Read the model definition and answer for the solid it produces. Units are mm, in the model's axes. A direction names the side the tool comes from. Coordinates: 2 decimals unless noted, no trailing zeros. Order: outer loops, then holes, each group sorted by start corner. A loop starts at its lowest first (then second) coordinate and runs counter-clockwise, first axis right, second up. Notation, with made-up numbers: (29, 33) -> (72, 33) arc R28 ccw to (72, 52) -> close; hole circle Ø7 at (30.25, -19). An arc over 180 degrees is marked (long way). Answer in a Markdown table with one row per item.
from build123d import *

# Parameters (mm, degrees)
SKETCH100_R             = 17.579923
SKETCH100_R_2           = 1.617669
PAD044_DEPTH            = 8
SKETCH101_W             = 5
SKETCH101_H             = 3
SKETCH102_R             = 12.788983
SKETCH102_R_2           = 6.518589
POCKET072_DEPTH         = 2
SKETCH103_W             = 7.319854
SKETCH103_H             = 4.413105
POCKET073_DEPTH         = 8.001
POCKET075_DEPTH         = 108.636829
POLARPATTERN003_COUNT   = 7
SKETCH112_R             = 2
POCKET079_DEPTH         = 17
BODY019_PLACEMENT_ANGLE = 180


with BuildPart() as part:
    # Sketch100 → Pad044 (new body)
    with BuildSketch(Plane.YZ):
        Circle(SKETCH100_R)
        Circle(SKETCH100_R_2, mode=Mode.SUBTRACT)
    extrude(amount=PAD044_DEPTH)

    # Sketch101 → Groove003 (revolve, cut)
    with BuildSketch(Plane.XY):
        with Locations((4, 16.079923)):
            Rectangle(SKETCH101_W, SKETCH101_H)
    revolve(axis=Axis((0, 0, 0), (1, 0, 0)), mode=Mode.SUBTRACT)

    # Sketch102 (on Face6 of Groove003) → Pocket072 (cut)
    with BuildSketch(Plane.YZ.offset(8)):
        Circle(SKETCH102_R)
        Circle(SKETCH102_R_2, mode=Mode.SUBTRACT)
    extrude(amount=-POCKET072_DEPTH, mode=Mode.SUBTRACT)

    # Sketch103 (on Face11 of Pocket072) → Pocket073 (cut, through all)
    with BuildSketch(Plane.YZ.offset(8)):
        with Locations((-0.062492, 19.721895)):
            Rectangle(SKETCH103_W, SKETCH103_H)
    extrude(amount=-POCKET073_DEPTH, mode=Mode.SUBTRACT)

    # Sketch105 → Pocket075 (cut, through all)
    with BuildSketch(Plane.YZ.offset(8)):
        with BuildLine():
            ThreePointArc((4.568379, 12.912664), (0, 13.69697), (-4.568379, 12.912664))
            Line((-4.568379, 12.912664), (0, 5))
            Line((4.568379, 12.912664), (0, 5))
        make_face()
    pocket075 = extrude(amount=-POCKET075_DEPTH, mode=Mode.SUBTRACT)

    # PolarPattern003: Pocket075 ×7 about axis
    polarpattern003_axis = Axis((0, 0, 0), (1, 0, 0))
    for i in range(1, POLARPATTERN003_COUNT):
        add(pocket075.rotate(polarpattern003_axis, i * 360 / POLARPATTERN003_COUNT), mode=Mode.SUBTRACT)

    # Sketch112 (on Face55 of PolarPattern003) → Pocket079 (cut)
    with BuildSketch(Plane(origin=(0, 0, 17.515343), x_dir=(0, -1, 0), z_dir=(0, 0, 1))):
        with Locations((0, 4)):
            Circle(SKETCH112_R)
    extrude(amount=-POCKET079_DEPTH, mode=Mode.SUBTRACT)


with BuildPart() as part_1:
    # Body016 placement: moved
    add(part.part.moved(Location((46, 73, 0))))


with BuildPart() as part_2:
    # Body019 placement: moved
    add(part_1.part.rotate(Axis((0, 0, 0), (0, 1, 0)), BODY019_PLACEMENT_ANGLE))


solid = part_2.part
Q1. For a pull along X with two mould halves and no side action, classify faces 1 (the face through (-52, 80, 6)), 2 (the face through (-53.014, 67.885, 4.041)), 3 (the face through (-52.5, 83.5, 10.35)) as pulls with the +X half, pulls with the -X half, needs draft (parallel to the pull), parting line crosses it, or undercut.
Outcome:
| item | result |
|---|---|
| face 1 | pulls with the -X half |
| face 2 | needs draft |
| face 3 | undercut |
Q2. The part is cut by section A-A (z = 8). Write down the section's boundary in (x, y), then the cut area to 3 significant figures.
Outcome:
| item | result |
|---|---|
| outline | (-54, 57.35) -> (-52.5, 57.35) -> (-52.5, 60.81) -> (-47.5, 60.81) -> (-47.5, 57.35) -> (-46, 57.35) -> (-46, 65.7) -> (-52, 65.7) -> (-52, 63.02) -> (-54, 63.02) -> close; (-54, 82.98) -> (-52, 82.98) -> (-52, 80.3) -> (-46, 80.3) -> (-46, 88.65) -> (-47.5, 88.65) -> (-47.5, 85.19) -> (-52.5, 85.19) -> (-52.5, 88.65) -> (-54, 88.65) -> close; (-52, 71.09) -> (-46, 71.09) -> (-46, 74.91) -> (-52, 74.91) -> close |
| area | 111 mm² |
Q3. Given pin 1 (3 mm diameter, centred on y = 73, z = 0, fed in from +X); pin 2 (10 mm diameter, centred on y = 61, z = -13.5, fed in from +X); pin 3 (3 mm diameter, centred on x = -51.5, y = 75.5, fed in from +Z); pin 4 (2.5 mm diameter, centred on y = 83.5, z = -2, fed in from -X), each flat-ended and moving along its own axis, determine where each tip first touches the part or whether it passes through.
Outcome:
| item | result |
|---|---|
| pin 1 | through |
| pin 2 | x = -46 |
| pin 3 | z = 17.53 |
| pin 4 | x = -52 |
Q4. For faces 4 (the face through (-47.5, 83.5, 10.35)), 5 (the face through (-49.94, 72.65, 1.58)), 6 (the face through (-53.01, 62.99, 7.96)), determine the directions among +Z, -Z, +X, -X, +Y, -Y from which every point of the face is accessible in a straight line to the end or side of a thin tool.
Outcome:
| item | result |
|---|---|
| face 4 | none |
| face 5 | +X, -X |
| face 6 | -X |
Q5. The part is cut by section C-C (x = -50). Give the number of separate pieces and of enclosed holes in the cut face, then the cut area to 3 significant figures.
Outcome:
| item | result |
|---|---|
| separate pieces | 1 |
| enclosed holes | 6 |
| area | 347 mm² |
Q6. Consider line 1 (Z direction, x = -47, y = 69.5); line 2 (Y direction, x = -46.75, z = 11); line 3 (Y direction, x = -53, z = -2). Determine where each line is inside the solid, lowest interval first.
Outcome:
| item | result |
|---|---|
| line 1 | -17.23 to -13.24, -11.06 to 5.41, 13.24 to 17.23 |
| line 2 | 59.29 to 64.84, 71.32 to 74.68, 81.16 to 86.71 |
| line 3 | 55.53 to 60.37, 66.8 to 79.2, 85.63 to 90.47 |
Q7. The part is cut by section B-B (z = 0). Write down the section's boundary in (x, y).
Outcome:
| item | result |
|---|---|
| outline | (-54, 55.42) -> (-52.5, 55.42) -> (-52.5, 58.42) -> (-47.5, 58.42) -> (-47.5, 55.42) -> (-46, 55.42) -> (-46, 59.3) -> (-54, 59.3) -> close; (-54, 66.48) -> (-52, 66.48) -> (-52, 64.52) -> (-46, 64.52) -> (-46, 71.38) -> (-54, 71.38) -> close; (-54, 74.62) -> (-46, 74.62) -> (-46, 81.48) -> (-52, 81.48) -> (-52, 79.52) -> (-54, 79.52) -> close; (-54, 86.7) -> (-46, 86.7) -> (-46, 90.58) -> (-47.5, 90.58) -> (-47.5, 87.58) -> (-52.5, 87.58) -> (-52.5, 90.58) -> (-54, 90.58) -> close |
